Source: CAD feature listing. Evaluate the final solid. Frame: model axes, mm. A direction names the side the tool comes from. Round coordinates to 2 decimals unless told otherwise and drop trailing zeros. Loops run counter-clockwise (first coordinate to the right, second up) from the corner with the lowest first, then second, coordinate; pieces in that order, holes last. Notation, with made-up numbers: M -13.75,82 L 43.25,82 A25 ccw 43.25,118 Z; hole C 52,47 d3. An arc over 180 degrees is marked long. Write each question's results on one line, items separated by ' | '. Start each with the question number.
1. Section A-A on z = 3.25. Output: boundary loops of the cut face in (x, y) (3 decimals), and give its area (3 significant figures).
2. Ray query, line 1 (Z direction, x = 3, y = -5); line 2 (Y direction, x = 0, z = 3.75) (3 decimals); line 3 (Y direction, x = 0, z = 11.25) (3 decimals). Return the intervals inside material, ascending.
3. Section B-B on z = 6.5. Output: boundary loops of the cut face in (x, y) (3 decimals), and give its area (3 significant figures).
4. Draft query along Z for faces 1 (the cylindrical face through (0.69, -3.1, 7.84)), 2 (the flat face through (3.4, 0.1, 15.9)), 3 (the cylindrical face through (3.607, -3.849, 10.752)). Return one class per face: released by +Z, released by -Z, zero draft, split by the parting line, or undercut.
5. Contact query for flat-ended pins moving along their axis: pin 1 Ø2 at (x, y) = (6, 2) entering from -Z; pin 2 Ø2 at (y, z) = (2.5, 9) entering from -X; pin 3 Ø2 at (x, z) = (4.5, 7) entering from -Y; pin 4 Ø5 at (x, y) = (0, 0) entering from +Z. Output: stop coordinate, or through.
6. Set-up query: faces 4 (the cylindrical face through (-1.73, -7.81, 2.96)), 5 (the cylindrical face through (-3.607, 3.849, 10.752)). Return all of +Z, -Z, +X, -X, +Y, -Y with unobstructed straight access to the full face (end or side cutting, diameter ignored); none if empty.
from build123d import *

# Parameters (mm, degrees)
F0_R     = 8
F1_DEPTH = 7
F2_R     = 6
F3_DEPTH = 7.4
F4_SIZE  = 1
F5_R     = 8
F6_DEPTH = 1.5
F7_R     = 0.725
F8_DEPTH = 7.4
F10_D    = 6.35


with BuildPart() as f1:
    # F0 (on Top) → F1 (new body)
    with BuildSketch(Plane.XY):
        Circle(F0_R)
    extrude(amount=F1_DEPTH)

    # F2 (on face) → F3 (join)
    with BuildSketch(Plane.XY.offset(7)):
        Circle(F2_R)
    extrude(amount=F3_DEPTH)

    # F4
    f4_edges = [f1.edges().sort_by_distance(p)[0] for p in [
        (-8, 0, 7),
    ]]
    chamfer(f4_edges, length=F4_SIZE)

    # F5 (on face) → F6 (join)
    with BuildSketch(Plane.XY.offset(14.4)):
        Circle(F5_R)
    extrude(amount=F6_DEPTH)

    # F7 (on face) → F8 (cut)
    with BuildSketch(Plane(origin=(0, 0, 14.4), x_dir=(1, 0, 0), z_dir=(0, 0, -1))):
        with Locations((-5.4243303263, 2.5644961514)):
            Circle(F7_R)
        with Locations((-5.9513175962, 0.7627705219)):
            Circle(F7_R)
        with Locations((-5.8957484345, -1.1136204009)):
            Circle(F7_R)
        with Locations((-5.2630623379, -2.8810023997)):
            Circle(F7_R)
        with Locations((-4.1151910298, -4.3663718106)):
            Circle(F7_R)
        with Locations((-2.5644961514, -5.4243303263)):
            Circle(F7_R)
        with Locations((-0.7627705219, -5.9513175962)):
            Circle(F7_R)
        with Locations((1.1136204009, -5.8957484345)):
            Circle(F7_R)
        with Locations((2.8810023997, -5.2630623379)):
            Circle(F7_R)
        with Locations((4.3663718106, -4.1151910298)):
            Circle(F7_R)
        with Locations((5.4243303263, -2.5644961514)):
            Circle(F7_R)
        with Locations((5.9513175962, -0.7627705219)):
            Circle(F7_R)
        with Locations((5.8957484345, 1.1136204009)):
            Circle(F7_R)
        with Locations((5.2630623379, 2.8810023997)):
            Circle(F7_R)
        with Locations((4.1151910298, 4.3663718106)):
            Circle(F7_R)
        with Locations((2.5644961514, 5.4243303263)):
            Circle(F7_R)
        with Locations((0.7627705219, 5.9513175962)):
            Circle(F7_R)
        with Locations((-1.1136204009, 5.8957484345)):
            Circle(F7_R)
        with Locations((-2.8810023997, 5.2630623379)):
            Circle(F7_R)
        with Locations((-4.3663718106, 4.1151910298)):
            Circle(F7_R)
    extrude(amount=F8_DEPTH, mode=Mode.SUBTRACT)

    # F10 (through all)
    with Locations(Plane.XY.offset(15.9)):
        with Locations((0, 0)):
            Hole(F10_D / 2)


solid = f1.part
Taken from the geometry:
1) outline: C 0,0 d16; hole C 0,0 d6.35 | area: 169 mm^2
2) line 1: 0 to 7, 14.4 to 15.9 | line 2: -8 to -3.175, 3.175 to 8 | line 3: -6 to -3.175, 3.175 to 6
3) outline: C 0,0 d15; hole C 0,0 d6.35 | area: 145 mm^2
4) face 1: zero draft | face 2: released by +Z | face 3: undercut
5) pin 1: z = 0 | pin 2: x = -5.72 | pin 3: y = -6.77 | pin 4: through
6) face 4: +Z, -Z | face 5: none
